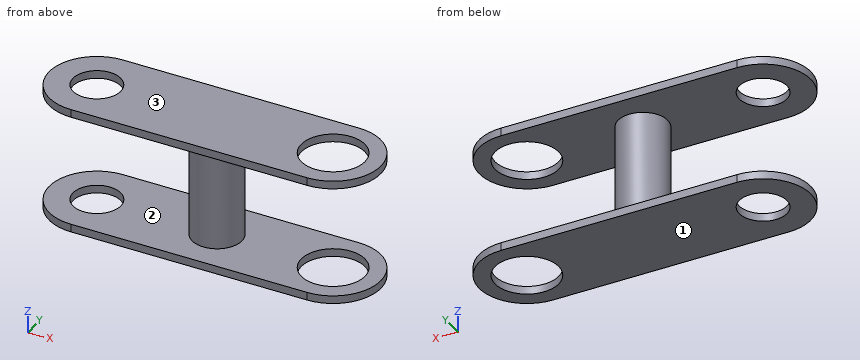
from build123d import *

# Parameters (mm, degrees)
SKETCH_1_R             = 15
SKETCH_1_R_2           = 20
EXTRUDE_1_DEPTH        = 5
SKETCH_2_R             = 15.619945806
EXTRUDE_2_DEPTH        = 70
PATTERN_LINEAR_1_COUNT = 2
PATTERN_LINEAR_1_PITCH = 75


with BuildPart() as part:
    # 草图1 → 凸台-拉伸1 (new body)
    with BuildSketch(Plane.XY):
        with BuildLine():
            Line((-31.598747919, 30), (118.401252081, 30))
            ThreePointArc((118.401252081, 30), (148.401252081, 0), (118.401252081, -30))
            Line((118.401252081, -30), (-31.598747919, -30))
            ThreePointArc((-31.598747919, -30), (-61.598747919, 0), (-31.598747919, 30))
        make_face()
        with Locations((-31.598747919, 0)):
            Circle(SKETCH_1_R, mode=Mode.SUBTRACT)
        with Locations((118.401252081, 0)):
            Circle(SKETCH_1_R_2, mode=Mode.SUBTRACT)
    extrude_1 = extrude(amount=EXTRUDE_1_DEPTH)

    # 草图2 → 凸台-拉伸2 (add)
    with BuildSketch(Plane.XY.offset(5)):
        with Locations((44.713404219, 0)):
            Circle(SKETCH_2_R)
    extrude(amount=EXTRUDE_2_DEPTH)

    # 阵列(线性)1: 凸台-拉伸1 ×2
    with Locations(*[(0, 0, i * PATTERN_LINEAR_1_PITCH) for i in range(1, PATTERN_LINEAR_1_COUNT)]):
        add(extrude_1)


solid = part.part
Model file for the job. Use its own axes, mm. Face numbers are marked on the shaded views. Give positions to 0.01 mm unless a question says otherwise; leave off trailing zeros. Order: outer loops, then holes, each group sorted by start corner. A loop starts at its lowest first (then second) coordinate and runs counter-clockwise, first axis right, second up. Notation, with made-up numbers: (7.25, 12) - (43.25, 12) arc R8 ccw to (43.25, 19) - close; hole circle Ø3 at (-21, -16). An arc over 180 degrees is marked (long way). Return JSON: item names as keys, results as strings.
1) Probe line 1 (Z direction, x = 54.5, y = 13); line 2 (X direction, y = -4.5, z = 21.5); line 3 (X direction, y = -8.5, z = 16). List the from-to ranges inside material, lowest first. Write a range as from..to.
Geometry says:
{"line 1": "0..5, 75..80", "line 2": "29.76..59.67", "line 3": "31.61..57.82"}
2) Pull direction Z, two halves, no side cores. Call the marked faces 1, 2 and 3: pulls with the +Z half, pulls with the -Z half, needs draft (parallel to the pull), parting line crosses it, or undercut.
Geometry says:
{"face 1": "pulls with the -Z half", "face 2": "undercut", "face 3": "pulls with the +Z half"}
3) Cut at B-B, the plane y = 0. Give the cut face in (x, z), plus the area to 3 significant figures.
Geometry says:
{"outline": "(-61.6, 0) - (-46.6, 0) - (-46.6, 5) - (-61.6, 5) - close; (-61.6, 75) - (-46.6, 75) - (-46.6, 80) - (-61.6, 80) - close; (-16.6, 0) - (98.4, 0) - (98.4, 5) - (60.33, 5) - (60.33, 75) - (98.4, 75) - (98.4, 80) - (-16.6, 80) - (-16.6, 75) - (29.09, 75) - (29.09, 5) - (-16.6, 5) - close; (138.4, 0) - (148.4, 0) - (148.4, 5) - (138.4, 5) - close; (138.4, 75) - (148.4, 75) - (148.4, 80) - (138.4, 80) - close", "area": "3,590 mm²"}
4) Cut at A-A, the plane x = 26.5. Give the cut face in (y, z).
Geometry says:
{"outline": "(-30, 0) - (30, 0) - (30, 5) - (-30, 5) - close; (-30, 75) - (30, 75) - (30, 80) - (-30, 80) - close"}
5) Flat gauge pins, fed straight in: P1, Ø5, axis at y = -2.5, z = 58.5, coming from the -X side; P2, Ø24, axis at x = -31.6, y = 0, coming from the +Z side; P3, Ø10, axis at x = 58.5, z = 27.5, coming from the -Y side; P4, Ø8, axis at y = 14, z = 36.5, coming from the -X side. Where does each tip first touch, or does it go through?
Geometry says:
{"P1": "x = 29.09", "P2": "through", "P3": "y = -12.91", "P4": "x = 32.71"}
6) Cut at C-C, the plane z = 38. Give the cut face in (x, y), plus the area to 3 significant figures.
Geometry says:
{"outline": "circle Ø31.24 at (44.71, 0)", "area": "766 mm²"}
